Here's how the part is built. I have some questions about the finished solid (model axes, mm). Face numbers are marked on the shaded views. A direction names the side the tool comes from. Give positions to 0.01 mm unless a question says otherwise; leave off trailing zeros. Loops run counter-clockwise (first coordinate to the right, second up) from the corner with the lowest first, then second, coordinate; pieces in that order, holes last. Notation, with made-up numbers: (45.5, 40) - (70.5, 40) arc R10 ccw to (70.5, 45) - close; hole circle Ø2 at (-2, 9). An arc over 180 degrees is marked (long way). Return JSON: item names as keys, results as strings. Group by question number.
(1) If we section it at A-A (z = 12): Please give me the cut outline in (x, y), then the cut area to 3 significant figures.
(2) On a 3-axis mill with a long thin cutter (end or side, diameter ignored), from which of +Z, -Z, +X, -X, +Y, -Y can I reach the whole of each face in a straight line? I mean the marked faces 1 and 2. Say none if no direction works.
(3) I need wall thicknesses on probe 1 along X at (y, z) = (4.5, 26.25); probe 2 along Y at (x, z) = (18.5, 7.25); probe 3 along Z at (x, y) = (6.5, 0). Which ranges of each line are inside material? Lowest first, please. Write a range as [from, to].
(4) If we mould it in two halves opening along Y, with no side actions, what happens to the marked faces 3, 4 and 5? For each: released by +Y, released by -Y, zero draft, split by the parting line, or undercut.
(5) If we section it at B-B (y = 1): Please give me the cut outline in (x, z), then the cut area to 3 significant figures.
(6) For P1, Ø12, axis at x = 2, y = 6.5, coming from the +Z side, with a flat end and sliding along its axis, tell me the tip position at first contact or that it passes through.
(7) If we section it at C-C (x = -3): Please give me the cut outline in (y, z).
```python
from build123d import *

# Parameters (mm, degrees)
F0_W     = 45.500002
F0_H     = 45.500004
F0_W_2   = 41.416668
F0_H_2   = 41.027776
F1_DEPTH = 2
F2_DEPTH = 30
F3_R     = 2


with BuildPart() as f1:
    # F0 (on Top) → F1 (new body)
    with BuildSketch(Plane.XY):
        with Locations((0.291666, -0.097222)):
            Rectangle(F0_W, F0_H)
        Rectangle(F0_W_2, F0_H_2, mode=Mode.SUBTRACT)
        Rectangle(F0_W_2, F0_H_2)
    extrude(amount=F1_DEPTH)

    # F0 (on Top) → F2 (join)
    with BuildSketch(Plane.XY):
        with Locations((0.291666, -0.097222)):
            Rectangle(F0_W, F0_H)
        Rectangle(F0_W_2, F0_H_2, mode=Mode.SUBTRACT)
    extrude(amount=F2_DEPTH)

    # F3
    f3_edges = [f1.edges().sort_by_distance(p)[0] for p in [
        (-22.458335, -22.847224, 15),
        (23.041667, -22.847224, 15),
        (23.041667, 22.65278, 15),
        (-22.458335, 22.65278, 15),
    ]]
    fillet(f3_edges, radius=F3_R)


solid = f1.part
```
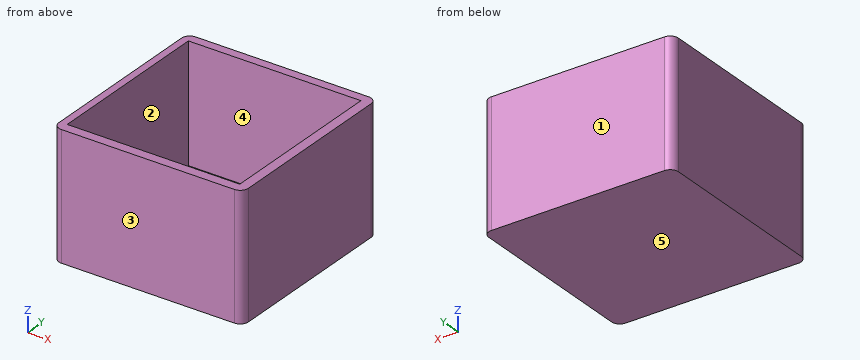
Values:
{
 "1": {"outline": "(-22.46, -20.85) arc R2 ccw to (-20.46, -22.85) - (21.04, -22.85) arc R2 ccw to (23.04, -20.85) - (23.04, 20.65) arc R2 ccw to (21.04, 22.65) - (-20.46, 22.65) arc R2 ccw to (-22.46, 20.65) - close; hole (-20.71, -20.51) - (20.71, -20.51) - (20.71, 20.51) - (-20.71, 20.51) - close", "area": "368 mm2"},
 "2": {"face 1": "+Z, -Z, +X, -X, +Y", "face 2": "+Z"},
 "3": {"probe 1": "[-22.46, -20.71], [20.71, 23.04]", "probe 2": "[-22.85, -20.51], [20.51, 22.65]", "probe 3": "[0, 2]"},
 "4": {"face 3": "released by -Y", "face 4": "undercut", "face 5": "zero draft"},
 "5": {"outline": "(-22.46, 0) - (23.04, 0) - (23.04, 30) - (20.71, 30) - (20.71, 2) - (-20.71, 2) - (-20.71, 30) - (-22.46, 30) - close", "area": "205 mm2"},
 "6": {"P1": "z = 2"},
 "7": {"outline": "(-22.85, 0) - (22.65, 0) - (22.65, 30) - (20.51, 30) - (20.51, 2) - (-20.51, 2) - (-20.51, 30) - (-22.85, 30) - close"}
}
